Geometry check sheet. Reference: the model listing, model coordinates, mm. Coordinates: 2 decimals unless noted, no trailing zeros. Loops run counter-clockwise (first coordinate to the right, second up) from the corner with the lowest first, then second, coordinate; pieces in that order, holes last. Notation, with made-up numbers: (33, 23) -> (62, 23) arc R19 ccw to (62, 52) -> close; hole circle Ø3 at (-8.75, -20). An arc over 180 degrees is marked (long way). Answer as a JSON object with one key per item and string values.
from build123d import *

# Parameters (mm, degrees)
BOSS_EXTRUDE1_DEPTH = 4.3


with BuildPart() as part:
    # Sketch1 → Boss-Extrude1 (new body)
    with BuildSketch(Plane(origin=(0, 0, 0), x_dir=(0, 0, -1), z_dir=(1, 0, 0))):
        with BuildLine():
            Line((10.377941535, 10.968515373), (24.883087867, 4.215684123))
            ThreePointArc((24.883087867, 4.215684123), (24.37551983, 3.75), (23.687326628, 3.7796164))
            Line((23.687326628, 3.7796164), (9.577602267, 10.348360032))
            ThreePointArc((9.577602267, 10.348360032), (9.104252866, 10.361422213), (8.647588121, 10.236172121))
            ThreePointArc((8.647588121, 10.236172121), (-0.351285356, 13.395394679), (-9.172206838, 9.768859797))
            Line((-9.172206838, 9.768859797), (-10.349710711, 10.995157488))
            ThreePointArc((-10.349710711, 10.995157488), (0.019408643, 15.099987527), (10.377941535, 10.968515373))
        make_face()
    extrude(amount=BOSS_EXTRUDE1_DEPTH)


solid = part.part
1. Section check A-A, the plane x = 2.7. Record the boundary of the cut face in (y, z).
Evaluation:
{"outline": "(3.78, -23.69) arc R0.9 ccw to (4.22, -24.88) -> (10.97, -10.38) arc R15.1 ccw to (11, 10.35) -> (9.77, 9.17) arc R13.4 cw to (10.24, -8.65) arc R1.61 cw to (10.35, -9.58) -> close"}
2. Section check D-D, the plane y = 14. Record the boundary of the cut face in (x, z), then the cut area to 3 significant figures.
Evaluation:
{"outline": "(0, -5.66) -> (4.3, -5.66) -> (4.3, 5.66) -> (0, 5.66) -> close", "area": "48.7 mm^2"}
3. Thickness scan on probe 1 along Z at (x, y) = (1.4, 11.25); probe 2 along Z at (x, y) = (2.2, 10.5); probe 3 along Y at (x, z) = (2.8, -19). Record the ranges inside material, lowest first. Write a range as from..to.
Evaluation:
{"probe 1": "z = -10.07..-7.28, 7.28..10.07", "probe 2": "z = -11.38..-8.33, 8.33..9.87", "probe 3": "y = 5.96..6.95"}
4. Section check C-C, the plane z = 2. Record the boundary of the cut face in (x, y), then the cut area to 3 significant figures.
Evaluation:
{"outline": "(0, 13.25) -> (4.3, 13.25) -> (4.3, 14.97) -> (0, 14.97) -> close", "area": "7.38 mm^2"}
5. Depth check by flat-ended pin: P1, Ø3, axis at y = 10, z = -5.5, coming from the -X side; P2, Ø1.5, axis at x = 1.5, y = 9.5, coming from the +Z side. Enter the tip coordinate at first touch or a pass-through.
Evaluation:
{"P1": "passes through", "P2": "stops at z = 9.63"}
6. Mould release check, pull along Z, two halves, no side actions. Record for faces 1 (the face through (2.12, 7.64, -17.53)), 2 (the face through (2.12, 10.362, -9.111)), 3 (the face through (0, 12.4, -6)), 4 (the face through (2.1, 15.1, 0.1)): released by +Z, released by -Z, zero draft, split by the parting line, or undercut.
Evaluation:
{"face 1": "released by -Z", "face 2": "undercut", "face 3": "zero draft", "face 4": "split by the parting line"}
7. Section check B-B, the plane y = 12. Record the boundary of the cut face in (x, z).
Evaluation:
{"outline": "(0, -9.17) -> (4.3, -9.17) -> (4.3, -5.96) -> (0, -5.96) -> close; (0, 5.96) -> (4.3, 5.96) -> (4.3, 9.17) -> (0, 9.17) -> close"}
